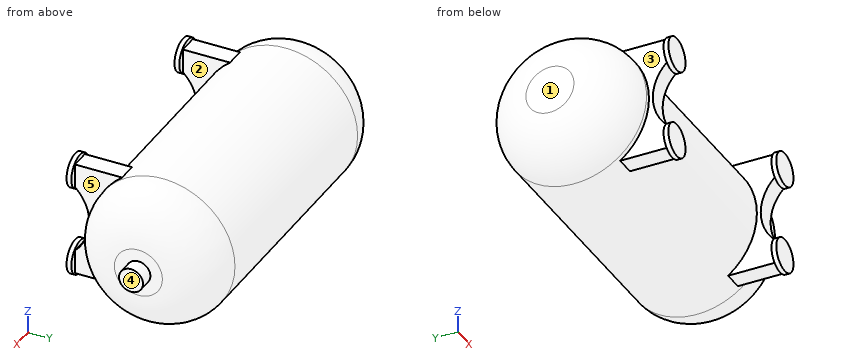
Autodesk Inventor part; units mm, degrees
ref_plane "YZ Plane" through (0, 0, 0) normal (1, 0, 0) x (0, 1, 0)
ref_plane "XZ Plane" through (0, 0, 0) normal (0, 1, 0) x (-1, 0, 0)
ref_plane "XY Plane" through (0, 0, 0) normal (0, 0, 1) x (1, 0, 0)
sketch "Sketch2" plane through (0, 0, 0) normal (1, 0, 0) x (0, 1, 0)
  circle A0 centre (0, 0) radius 75
  dimension "d2" = 150
extrude "Extrusion1" add sketch "Sketch2" along normal mid plane 350
fillet "Fillet1" radius 50 2 edges at (-175, -75, 0) (175, -75, 0)
sketch "Sketch3" plane through (175, 0, 0) normal (1, 0, 0) x (0, 0, -1)
  circle A0 centre (0, 0) radius 12.5
  dimension "d6" = 25
extrude "Extrusion2" add sketch "Sketch3" along normal blind 15
sketch "Sketch4" plane through (0, 0, 0) normal (0, 1, 0) x (-1, 0, 0)
  line L0 (120, 60) -> (100, 60)
  line L1 (100, 60) -> (100, -60)
  line L2 (100, -60) -> (120, -60)
  line L3 (120, -60) -> (120, 60)
  line L4 (120, 60) -> (100, -60) construction
  line L5 (100, 60) -> (120, -60) construction
  point P0 (0, 0)
  point P1 (110, 0)
  dimension "d9" = 20
  dimension "d10" = 120
extrude "Extrusion3" add sketch "Sketch4" against normal blind 94
mirror "Mirror1" about plane through (0, 0, 0) normal (1, 0, 0) of "Extrusion3"
sketch "Sketch5" plane through (-120, -94, -60) normal (-1, 0, 0) x (0, 0, 1)
  line L0 (0, 0) -> (120, 0)
  line L1 (0, 0) -> (25, 0)
  line L2 (25, 0) -> (25, 15)
  line L3 (25, 15) -> (0, 15)
  line L4 (0, 15) -> (0, 0)
  line L5 (95, 15) -> (120, 15)
  line L6 (120, 15) -> (120, 0)
  line L7 (120, 0) -> (95, 0)
  line L8 (95, 0) -> (95, 15)
  arc A0 (95, 0) -> (25, 0) centre (60, -33.3333) ccw
  line L9 (25, 0) -> (95, 0)
  point P0 (60, 94)
  dimension "d13" = 25
  dimension "d14" = 15
  dimension "d15" = 25
extrude "Extrusion4" cut sketch "Sketch5" against normal up to surface (240 mm away) contours A0 L0
sketch "Sketch7" plane through (0, -94, 0) normal (0, -1, 0) x (1, 0, 0)
  line L0 (-120, 35) -> (-100, 35)
  line L1 (-100, 35) -> (-100, 60)
  line L2 (-100, 60) -> (-120, 60)
  line L3 (-120, 60) -> (-120, 35)
  circle A0 centre (-110, 47.5) radius 17.5
  point P0 (0, 0)
  dimension "d18" = 35
extrude "Extrusion5" add sketch "Sketch7" along normal blind 5 contours L3 L2 L1 L0 | A0
mirror "Mirror2" about plane through (0, 0, 0) normal (0, 0, 1) of "Extrusion5"
mirror "Mirror3" about plane through (0, 0, 0) normal (1, 0, 0) of "Extrusion5", "Mirror2"
equation "\"d15\" = d13"
equation "\"BendRadius\" = Thickness"
equation "\"BendReliefWidth\" = Thickness"
equation "\"BendReliefDepth\" = 0.5 * Thickness"
equation "\"CornerReliefSize\" = 4 * Thickness"
equation "\"MinimumRemnant\" = 2 * Thickness"
equation "\"TransitionRadius\" = BendRadius"
equation "\"JacobiRadiusSize\" = BendRadius"
equation "\"GapSize\" = Thickness"
For this review, take the finished solid that the model builds, in its own axes (mm). Face numbers are marked on the shaded views. A direction names the side the tool comes from. Coordinates: 2 decimals unless noted, no trailing zeros. Loops run counter-clockwise (first coordinate to the right, second up) from the corner with the lowest first, then second, coordinate; pieces in that order, holes last. Notation, with made-up numbers: (-25.5, -15) -> (15.5, -15) arc R21 ccw to (15.5, -5) -> close; hole circle Ø8 at (16, 7). An arc over 180 degrees is marked (long way). Write each question's results on one line, items separated by ' | '.
Q1. To check wall thickness, follow line 1 along Y through (x, z) = (-24.5, -59); line 2 along Y through (x, z) = (-96.5, 22); line 3 along X through (y, z) = (49, -4.5). State the ranges of each line that lie inside material, in increasing order. Write a range as [from, to].
Taken from the geometry:
line 1: [-46.3, 46.3] | line 2: [-71.7, 71.7] | line 3: [-168.75, 168.75]
Q2. Machinability: for the marked faces 1, 2 and 3, which of the approach directions +Z, -Z, +X, -X, +Y, -Y give a long, thin tool a straight path to every point of the face, cutting with its end or side? Answer none if there is none.
Taken from the geometry:
face 1: +Z, -Z, -X, +Y, -Y | face 2: none | face 3: -X
Q3. Add section A-A, the plane x = -110. State the section outline as (y, z) points.
Taken from the geometry:
outline: (-99, -65) -> (-94, -65) -> (-94, -60) -> (-45, -60) arc R75 ccw (long way) to (-45, 60) -> (-94, 60) -> (-94, 65) -> (-99, 65) -> (-99, 30) -> (-94, 30) -> (-94, 35) arc R48.33 cw to (-94, -35) -> (-94, -30) -> (-99, -30) -> close
Q4. Add section B-B, the plane x = 66. State the section outline as (y, z) points, then the cut area to 3 significant figures.
Taken from the geometry:
outline: circle Ø150 at (0, 0) | area: 17,700 mm²
Q5. Mouldability with a two-part tool opening along Y and no side actions: class the marked faces 4 and 5 as +Y half, -Y half, draft (parallel to the pull), parting line (faces both ways), or undercut.
Taken from the geometry:
face 4: draft | face 5: undercut
Q6. For pin 1 Ø10.5 at (x, z) = (-109.5, 43) entering from +Y; pin 2 Ø1 at (x, z) = (77.5, -55.5) entering from -Y; pin 3 Ø14.5 at (y, z) = (-67.5, 15.5) entering from +X, all flat-tipped, find the tip position at first contact; note any pin that passes through.
Taken from the geometry:
pin 1: y = 64.81 | pin 2: y = -50.99 | pin 3: x = 158.62
